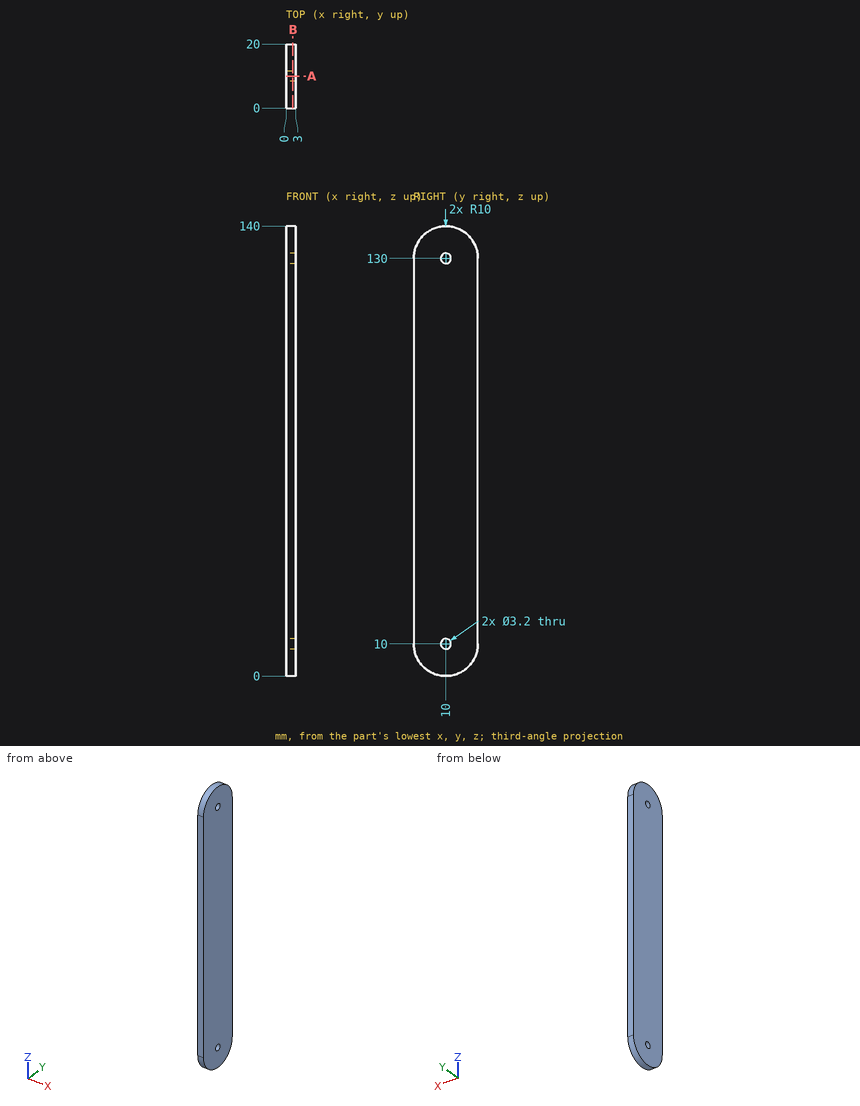
The drawing under review shows one solid part. Ordinate dimensions are in mm from its lowest x, y, z. Give positions to 0.01 mm unless a question says otherwise; leave off trailing zeros. Order: outer loops, then holes, each group sorted by start corner. A loop starts at its lowest first (then second) coordinate and runs counter-clockwise, first axis right, second up. Notation, with made-up numbers: (48, -22.5) - (65, -22.5) arc R19 ccw to (65, 13.5) - close; hole circle Ø8 at (-23.75, 83.25). An arc over 180 degrees is marked (long way). Answer as a JSON object with one key per item and string values. Group by question number.
Item 1: Take a section at B-B on x = 2.1. Give the boundary of the cut face in (y, z), and give its area (3 significant figures).
Item 2: Wall thickness on line 1 along Z through (x, y) = (1.2, 10); line 2 along Y through (x, z) = (2.15, 130); line 3 along Z through (x, y) = (1.3, 11.25): over which ranges is each line inside the solid? List them lowest first.
Item 3: Take a section at A-A on y = 10. Give the boundary of the cut face in (x, z).
Reported:
{
 "1": {"outline": "(0, 10) arc R10 ccw to (20, 10) - (20, 130) arc R10 ccw to (0, 130) - close; hole circle Ø3.2 at (10, 10); hole circle Ø3.2 at (10, 130)", "area": "2,700 mm^2"},
 "2": {"line 1": "0 to 8.4, 11.6 to 128.4, 131.6 to 140", "line 2": "0 to 8.4, 11.6 to 20", "line 3": "0.08 to 9, 11 to 129, 131 to 139.92"},
 "3": {"outline": "(0, 0) - (3, 0) - (3, 8.4) - (0, 8.4) - close; (0, 11.6) - (3, 11.6) - (3, 128.4) - (0, 128.4) - close; (0, 131.6) - (3, 131.6) - (3, 140) - (0, 140) - close"}
}
